```python
from build123d import *


with BuildPart() as f1:
    # F0 (on Front) → F1 (revolve)
    with BuildSketch(Plane.XZ):
        with BuildLine():
            Line((0, 9), (0, 6))
            Line((0, 6), (18.993515, 6))
            ThreePointArc((18.993515, 6), (23.252285, 4.790172), (26.238968, 1.522063))
            Line((26.238968, 1.522063), (27, 0))
            Line((27, 0), (30, 0))
            Line((30, 0), (37.42918, 12.974822))
            ThreePointArc((37.42918, 12.974822), (38.227719, 14.917411), (38.5, 17))
            Line((38.5, 17), (38.5, 18))
            Line((38.5, 18), (40.5, 18))
            Line((40.5, 18), (33.068382, 88.707122))
            ThreePointArc((33.068382, 88.707122), (32.59362, 89.581524), (31.639617, 89.864113))
            Line((31.639617, 89.864113), (31.241808, 89.822302))
            ThreePointArc((31.241808, 89.822302), (30.367405, 89.34754), (30.084816, 88.393536))
            Line((30.084816, 88.393536), (37.111707, 21.537138))
            ThreePointArc((37.111707, 21.537138), (36.982068, 19.020359), (36.085263, 16.66521))
            Line((36.085263, 16.66521), (34.029843, 13.075486))
            ThreePointArc((34.029843, 13.075486), (31.062889, 10.092548), (27, 9))
            Line((27, 9), (0, 9))
        make_face()
    revolve(axis=Axis((0, 0, 44.353561), (0, 0, 1)))


solid = f1.part
```
Geometry: final body of the model. Coordinates: model frame, mm. A direction names the side the tool comes from. Give positions to 0.01 mm unless a question says otherwise; leave off trailing zeros. Write each loop counter-clockwise with the first axis right and the second up, starting at its lowest first coordinate (ties: lowest second). Pieces come first, ordered by that corner, then holes.
1. Reachability of faces 4 (the conical face through (-7.29, -32.85, 54.5)), 5 (the flat face through (-36, -15, 18)), 6 (the flat face through (0, 0, 9)) from +Z, -Z, +X, -X, +Y, -Y: full face, straight path, thin tool, end or side. Return the list, or none.
2. Pin query (flat end, axial travel): P1, Ø3, axis at y = -5, z = 80.5, coming from the -X side; P2, Ø1.5, axis at y = 27.5, z = 71, coming from the +X side; P3, Ø2, axis at x = 14, z = 9, coming from the +Y side. Return the tip coordinate at first contact, or that it passes through.
3. Section query C-C, the plane z = 64. Return loops of the section in (x, y).
4. Line query: probe 1 along Y at (x, z) = (-17, 73.5); probe 2 along X at (y, z) = (-12, 49.5); probe 3 along Z at (x, y) = (-6, -8). Output: solid intervals per line, ascending.
5. Section query D-D, the plane z = 27.5. Return loops of the section in (x, y), then the cut area to 3 significant figures.
6. Draft query along X for faces 1 (the conical face through (16.95, -32.588, 53.849)), 2 (the flat face through (25, 11, 0)), 3 (the flat face through (0, 0, 6)). Return one class per face: released by +X, released by -X, zero draft, split by the parting line, or undercut.
Computed:
1. face 4: none
1. face 5: -Z
1. face 6: +Z
2. P1: stops at x = -33.81
2. P2: stops at x = 22.47
2. P3: stops at y = 33
3. outline: circle Ø71.33 at (0, 0); hole circle Ø65.3 at (0, 0)
4. probe 1: y = -30.21 to -26.7, 26.7 to 30.21
4. probe 2: x = -35.2 to -32, 32 to 35.2
4. probe 3: z = 6 to 9
5. outline: circle Ø79 at (0, 0); hole circle Ø72.97 at (0, 0)
5. area: 720 mm2
6. face 1: split by the parting line
6. face 2: zero draft
6. face 3: undercut
